Build history of the part. All positions in model axes, mm. Round coordinates to 2 decimals unless told otherwise and drop trailing zeros. Loops run counter-clockwise (first coordinate to the right, second up) from the corner with the lowest first, then second, coordinate; pieces in that order, holes last.
from build123d import *

# Parameters (mm, degrees)
SKETCH1_R           = 12
BOSS_EXTRUDE1_DEPTH = 4
SKETCH3_R           = 1.5
CUT_EXTRUDE1_DEPTH  = 8
SKETCH4_R           = 2
CUT_EXTRUDE2_DEPTH  = 8
FILLET1_R           = 0.2


with BuildPart() as part:
    # Sketch1 → Boss-Extrude1 (new, symmetric)
    with BuildSketch(Plane.XY):
        Polygon((-14, 6), (-14, -6), (-6, -16), (6, -16), (14, -6), (14, 6), (6, 16), (-6, 16), align=None)
        Circle(SKETCH1_R, mode=Mode.SUBTRACT)
    extrude(amount=BOSS_EXTRUDE1_DEPTH, both=True)

    # Sketch2 → Cut-Revolve1 (revolve, cut)
    with BuildSketch(Plane.XY, mode=Mode.PRIVATE) as cut_revolve1_sk:
        Polygon((7.590491025, 7.590491025), (12.891478597, 12.891478597), (11.830818425, 13.952138769), (6.529830853, 8.651151197), align=None)
    revolve(cut_revolve1_sk.sketch.rotate(Axis((7.590491025, 7.590491025, 0), (0.7071067811865511, 0.707106781186544, 0)), 180), axis=Axis((7.590491025, 7.590491025, 0), (0.7071067811865511, 0.707106781186544, 0)), mode=Mode.SUBTRACT)

    # Sketch3 → Cut-Extrude1 (cut)
    with BuildSketch(Plane(origin=(0, 16, 0), x_dir=(1, 0, 0), z_dir=(0, 1, 0))):
        with Locations(Location((0, 0, 0), (0, 0, 270))):
            Circle(SKETCH3_R)
    extrude(amount=-CUT_EXTRUDE1_DEPTH, mode=Mode.SUBTRACT)

    # Sketch4 → Cut-Extrude2 (cut)
    with BuildSketch(Plane.XZ.offset(16)):
        with Locations(Location((0, 0, 0), (0, 0, 270))):
            Circle(SKETCH4_R)
    extrude(amount=-CUT_EXTRUDE2_DEPTH, mode=Mode.SUBTRACT)

    # Fillet1
    fillet1_edges = [part.edges().sort_by_distance(p)[0] for p in [
        (14, 0, -4),
        (10, -11, -4),
        (0, -16, -4),
        (-10, -11, -4),
        (10, -11, 4),
        (-14, -6, 0),
        (-14, 6, 0),
        (-6, 16, 0),
        (6, 16, 0),
        (14, 6, 0),
        (14, -6, 0),
        (6, -16, 0),
        (-6, -16, 0),
        (14, 0, 4),
        (10, 11, 4),
        (-12, 0, -4),
        (-12, 0, 4),
        (0, 16, 4),
        (-10, 11, 4),
        (-14, 0, 4),
        (-10, -11, 4),
        (-14, 0, -4),
        (0, -16, 4),
        (-10, 11, -4),
        (0, 16, -4),
        (10, 11, -4),
    ]]
    fillet(fillet1_edges, radius=FILLET1_R)


solid = part.part
(1) Slice it at B-B on y = 0. List the corners of the cut face in (x, z).
Responses:
outline: (-14, -3.8) arc R0.2 ccw to (-13.8, -4) - (-12.2, -4) arc R0.2 ccw to (-12, -3.8) - (-12, 3.8) arc R0.2 ccw to (-12.2, 4) - (-13.8, 4) arc R0.2 ccw to (-14, 3.8) - close; (12, -3.8) arc R0.2 ccw to (12.2, -4) - (13.8, -4) arc R0.2 ccw to (14, -3.8) - (14, 3.8) arc R0.2 ccw to (13.8, 4) - (12.2, 4) arc R0.2 ccw to (12, 3.8) - close
(2) Probe line 1 (Z direction, x = 0, y = 14.9); line 2 (Z direction, x = 0, y = -14.6); line 3 (X direction, y = 13.3, z = 0). List the from-to ranges inside material, lowest first.
Responses:
line 1: z = -4 to -1.5, 1.5 to 4
line 2: z = -4 to -2, 2 to 4
line 3: x = -8.16 to -1.5, 1.5 to 8.16
(3) Slice it at A-A on x = 0. List the corners of the cut face in (y, z).
Responses:
outline: (-16, -3.8) arc R0.2 ccw to (-15.8, -4) - (-12.2, -4) arc R0.2 ccw to (-12, -3.8) - (-12, -2) - (-16, -2) - close; (-16, 2) - (-12, 2) - (-12, 3.8) arc R0.2 ccw to (-12.2, 4) - (-15.8, 4) arc R0.2 ccw to (-16, 3.8) - close; (12, -3.8) arc R0.2 ccw to (12.2, -4) - (15.8, -4) arc R0.2 ccw to (16, -3.8) - (16, -1.5) - (12, -1.5) - close; (12, 1.5) - (16, 1.5) - (16, 3.8) arc R0.2 ccw to (15.8, 4) - (12.2, 4) arc R0.2 ccw to (12, 3.8) - close
(4) Pin check, flat tip, straight feed: P1, Ø1.5, axis at x = -10.5, z = -1.5, coming from the -Y side. Stop position of the tip, or through.
Responses:
P1: stops at y = -11.31
(5) Pull direction Y, two halves, no side cores. Call faces 1 (the face through (-10.02, 10.88, -3.94)), 2 (the face through (-11.99, 0.53, -0.05)), 3 (the face through (-2, -14, 0)): +Y half, -Y half, draft (parallel to the pull), parting line (faces both ways), or undercut.
Responses:
face 1: +Y half
face 2: undercut
face 3: draft
(6) Slice it at D-D on z = -1. List the corners of the cut face in (x, y).
Responses:
outline: (-14, -5.93) arc R0.2 ccw to (-13.96, -6.05) - (-6.06, -15.92) arc R0.2 ccw to (-5.9, -16) - (-1.73, -16) - (-1.73, -11.87) arc R12 cw to (-1.12, 11.95) - (-1.12, 16) - (-5.9, 16) arc R0.2 ccw to (-6.06, 15.92) - (-13.96, 6.05) arc R0.2 ccw to (-14, 5.93) - close; (1.12, 11.95) arc R12 cw to (7.66, 9.24) - (9.74, 11.32) - (6.06, 15.92) arc R0.2 ccw to (5.9, 16) - (1.12, 16) - close; (1.73, -16) - (5.9, -16) arc R0.2 ccw to (6.06, -15.92) - (13.96, -6.05) arc R0.2 ccw to (14, -5.93) - (14, 5.93) arc R0.2 ccw to (13.96, 6.05) - (11.15, 9.57) - (9.24, 7.66) arc R12 cw to (1.73, -11.87) - close
(7) Slice it at C-C on z = -3. List the corners of the cut face in (x, y), plus the area to 3 significant figures.
Responses:
outline: (-14, -5.93) arc R0.2 ccw to (-13.96, -6.05) - (-6.06, -15.92) arc R0.2 ccw to (-5.9, -16) - (5.9, -16) arc R0.2 ccw to (6.06, -15.92) - (13.96, -6.05) arc R0.2 ccw to (14, -5.93) - (14, 5.93) arc R0.2 ccw to (13.96, 6.05) - (6.06, 15.92) arc R0.2 ccw to (5.9, 16) - (-5.9, 16) arc R0.2 ccw to (-6.06, 15.92) - (-13.96, 6.05) arc R0.2 ccw to (-14, 5.93) - close; hole circle Ø24 at (0, 0)
area: 284 mm2
